Design review of the part built by this model. Coordinates are the model's own, in mm. A direction names the side the tool comes from. Round coordinates to 2 decimals unless told otherwise and drop trailing zeros. Order: outer loops, then holes, each group sorted by start corner. A loop starts at its lowest first (then second) coordinate and runs counter-clockwise, first axis right, second up. Notation, with made-up numbers: M 50,41.25 L 87,41.25 A15 cw 87,54.25 Z; hole C -26,17 d6. An arc over 180 degrees is marked long. Write each question's results on one line, items separated by ' | '. Start each with the question number.
Item 1: Take a section at A-A, the plane x = 0. Count the separate pieces of the cut face and the enclosed holes in it, plus the area to 3 significant figures.
Item 2: Machinability: for faces 1 (the cylindrical face through (12.932, -5.362, -107.36)), 2 (the cylindrical face through (-4.44, 4.07, 10.94)), 3 (the flat face through (12.4, 4.5, -125)), 4 (the flat face through (0, 0, -140)), which of the approach directions +Z, -Z, +X, -X, +Y, -Y give a long, thin tool a straight path to every point of the face, cutting with its end or side? Answer none if there is none.
Item 3: Wall thickness on line 1 (Y direction, x = 0, z = -81.5) (3 decimals); line 2 (X direction, y = 5, z = -18); line 3 (Y direction, x = 3, z = -100.5) (3 decimals): over which ranges is each line inside the solid? List them lowest first. Write a range as [from, to].
Item 4: The part is to be moulded in two halves that separate along Z. For faces 5 (the cylindrical face through (8.767, -16.856, -61.625)), 6 (the cylindrical face through (12.932, -5.362, -17.36)), 7 (the flat face through (-4.5, -12.4, 0)), say which applies: +Z half, -Z half, draft (parallel to the pull), parting line (faces both ways), or undercut.
Item 5: Take a section at C-C, the plane z = -33. Write out the cut boundary in (x, y), plus the area to 3 significant figures.
Item 6: Clearance check with flat-ended pins moving along their axes: pin 1 (10 mm diameter, centred on x = -13.5, y = 11.5, fed in from +Z); pin 2 (2 mm diameter, centred on y = 14.5, z = -6.5, fed in from -X); pin 3 (4 mm diameter, centred on x = 11.5, z = -65.5, fed in from -Y). State where each tip first meets the part, or that it passes through.
```python
from build123d import *

# Parameters (mm, degrees)
SKETCH1_R                 = 19
SKETCH1_R_2               = 14
BOSS_EXTRUDE1_DEPTH       = 125
BOSS_EXTRUDE2_START       = 7.5
SKETCH2_R                 = 14
BOSS_EXTRUDE2_DEPTH       = 7.5
CUT_EXTRUDE1_DEPTH        = 121.53319045
CUT_EXTRUDE1_DEPTH_BACK   = 121.53319045
SKETCH4_R                 = 6.025
SKETCH5_R                 = 14
BOSS_EXTRUDE3_DEPTH       = 7.5
BOSS_EXTRUDE4_DEPTH       = 15
BOSS_EXTRUDE4_DEPTH_BACK  = 140
SKETCH7_R                 = 6.025
SKETCH8_R                 = 15
BOSS_EXTRUDE5_DEPTH       = 5
LPATTERN2_COUNT           = 2
LPATTERN2_PITCH           = 30
LPATTERN3_COPY_1_SKETCH_R = 15
LPATTERN3_COPY_1_DEPTH    = 5
LPATTERN3_COPY_2_SKETCH_R = 15
LPATTERN3_COPY_2_DEPTH    = 5
FILLET1_R                 = 7


with BuildPart() as part:
    # Sketch1 → Boss-Extrude1 (new body)
    with BuildSketch(Plane.XY):
        Circle(SKETCH1_R)
        Circle(SKETCH1_R_2, mode=Mode.SUBTRACT)
    extrude(amount=-BOSS_EXTRUDE1_DEPTH)

    # Sketch2 → Boss-Extrude2 (add)
    with BuildSketch(Plane.XY.offset(-7.5).offset(BOSS_EXTRUDE2_START)):
        Circle(SKETCH2_R)
    extrude(amount=-BOSS_EXTRUDE2_DEPTH)

    # Sketch4 → Cut-Extrude1 (cut, two sides: drawn at the far end of the back side and taken through both)
    with BuildSketch(Plane.XY.offset(-7.5).offset(-CUT_EXTRUDE1_DEPTH_BACK)):
        Circle(SKETCH4_R)
    extrude(amount=CUT_EXTRUDE1_DEPTH + CUT_EXTRUDE1_DEPTH_BACK, mode=Mode.SUBTRACT)

    # Sketch5 → Boss-Extrude3 (add)
    with BuildSketch(Plane(origin=(0, 0, -117.5), x_dir=(-1, 0, 0), z_dir=(0, 0, -1))):
        with Locations(Location((0, 0, 0), (0, 0, 180))):
            Circle(SKETCH5_R)
    extrude(amount=BOSS_EXTRUDE3_DEPTH)

    # Sketch7 → Boss-Extrude4 (add, two sides: drawn at the far end of the back side and taken through both)
    with BuildSketch(Plane.XY.offset(-BOSS_EXTRUDE4_DEPTH_BACK)):
        Circle(SKETCH7_R)
    extrude(amount=BOSS_EXTRUDE4_DEPTH + BOSS_EXTRUDE4_DEPTH_BACK)

    # Sketch8 → Boss-Extrude5 (add, symmetric)
    with BuildSketch(Plane.XY.offset(-62.5)):
        Circle(SKETCH8_R)
    boss_extrude5 = extrude(amount=BOSS_EXTRUDE5_DEPTH, both=True)

    # LPattern2: Boss-Extrude5 ×2
    with Locations(*[(0, 0, -i * LPATTERN2_PITCH) for i in range(1, LPATTERN2_COUNT)]):
        add(boss_extrude5)

    # LPattern3 copy 1 sketch → LPattern3 copy 1 (add, symmetric)
    with BuildSketch(Plane.XY.offset(-62.5)):
        Circle(LPATTERN3_COPY_1_SKETCH_R)
    extrude(amount=LPATTERN3_COPY_1_DEPTH, both=True)

    # LPattern3 copy 2 sketch → LPattern3 copy 2 (add, symmetric)
    with BuildSketch(Plane.XY.offset(-32.5)):
        Circle(LPATTERN3_COPY_2_SKETCH_R)
    extrude(amount=LPATTERN3_COPY_2_DEPTH, both=True)

    # Fillet1
    fillet1_edges = [part.edges().sort_by_distance(p)[0] for p in [
        (-6.025, 0, 0),
        (-6.025, 0, -125),
    ]]
    fillet(fillet1_edges, radius=FILLET1_R)


solid = part.part
```
Results list:
1) separate pieces: 1 | enclosed holes: 8 | area: 3,880 mm²
2) face 1: none | face 2: +Z | face 3: -Z | face 4: -Z, +X, -X, +Y, -Y
3) line 1: [-19, -14], [-6.025, 6.025], [14, 19] | line 2: [-18.33, -13.08], [-3.36, 3.36], [13.08, 18.33] | line 3: [-18.762, -13.675], [-5.225, 5.225], [13.675, 18.762]
4) face 5: draft | face 6: undercut | face 7: +Z half
5) outline: C 0,0 d38 | area: 1,130 mm²
6) pin 1: z = 0.01 | pin 2: x = -13.37 | pin 3: y = -16.45
